Source: three-view drawing plus pictorial views. Frame: mm from the lowest corner of the part. A direction names the side the tool comes from. Round coordinates to 2 decimals unless told otherwise and drop trailing zeros. Loops run counter-clockwise (first coordinate to the right, second up) from the corner with the lowest first, then second, coordinate; pieces in that order, holes last. Notation, with made-up numbers: (13.25, -28.5) -> (55.25, -28.5) arc R9 cw to (55.25, -12.5) -> close; hole circle Ø1 at (12, -1). An arc over 180 degrees is marked (long way). One line per question, with ' | ' between items. Start each with the question number.
Q1. Cut plane D-D on x = 98. Return loops of the section in (y, z), and give its area (4 significant figures).
Q2. Contact query for flat-ended pins moving along their axis: P1, Ø3, axis at x = 62.5, y = 35, coming from the +Z side; P2, Ø11.5, axis at x = 27.5, z = 19.5, coming from the -Y side; P3, Ø3.5, axis at y = 22.5, z = 61.5, coming from the +X side. Output: stop coordinate, or through.
Q3. Cut plane C-C on y = 27. Return loops of the section in (x, z).
Q4. Material intervals for L1, parallel to Y at x = 65.5, z = 14; L2, parallel to X at y = 28, z = 55; L3, parallel to Y at x = 96, z = 70 (1 decimal), sorted ascending.
Q5. Access query for the marked faces 1, 2 and 3. Directions: +Z, -Z, +X, -X, +Y, -Y. A direction counts if a zero-diameter tool reaches every point of the face in a straight line with its end or side. Return the directions, or none.
Q6. Cut plane A-A on z = 21. Return loops of the section in (x, y).
Q7. Mould query, pull axis Y, two halves, no side actions, for the marked faces 4, 5 and 6. Classes: pulls with the +Y half, pulls with the -Y half, needs draft (parallel to the pull), parting line crosses it, or undercut.
Q8. Cut plane B-B on x = 55. Return loops of the section in (y, z) (1 decimal).
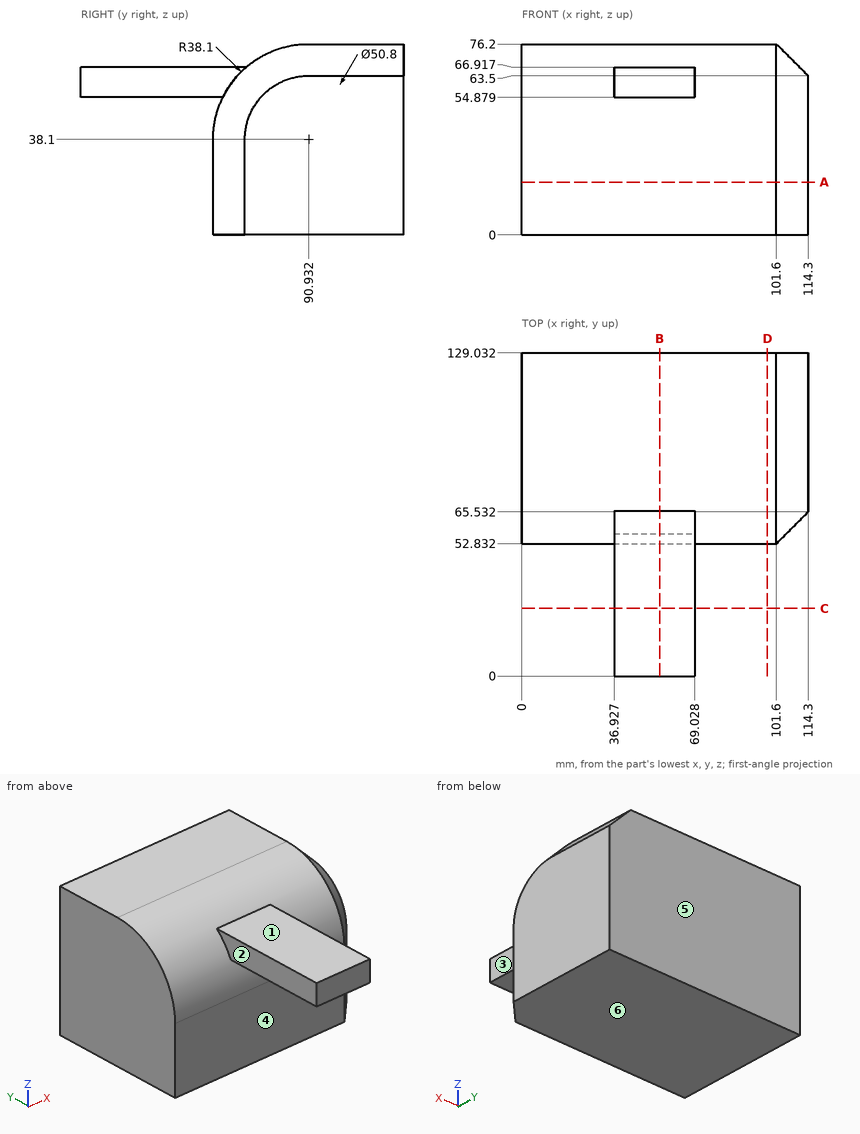
Results:
1) outline: (52.83, 0) -> (129.03, 0) -> (129.03, 76.2) -> (90.93, 76.2) arc R38.1 ccw to (52.83, 38.1) -> close | area: 5,495 mm^2
2) P1: z = 66.92 | P2: y = 52.83 | P3: x = 69.03
3) outline: (36.93, 54.88) -> (69.03, 54.88) -> (69.03, 66.92) -> (36.93, 66.92) -> close
4) L1: 52.83 to 129.03 | L2: 36.93 to 69.03 | L3: 70.1 to 129
5) face 1: +Z, +X, -X, -Y | face 2: +Z, -X, -Y | face 3: +Z, +X, -Y
6) outline: (0, 52.83) -> (101.6, 52.83) -> (114.3, 65.53) -> (114.3, 129.03) -> (0, 129.03) -> close
7) face 4: pulls with the -Y half | face 5: pulls with the +Y half | face 6: needs draft
8) outline: (0, 54.9) -> (56.7, 54.9) arc R38.1 ccw to (52.8, 38.1) -> (52.8, 0) -> (129, 0) -> (129, 76.2) -> (90.9, 76.2) arc R38.1 ccw to (66, 66.9) -> (0, 66.9) -> close
